Geometry check sheet. Reference: the model listing, model coordinates, mm. A direction names the side the tool comes from. Give positions to 0.01 mm unless a question says otherwise; leave off trailing zeros. Write each loop counter-clockwise with the first axis right and the second up, starting at its lowest first coordinate (ties: lowest second). Pieces come first, ordered by that corner, then holes. Notation, with made-up numbers: (11, 68) - (32, 68) arc R26 cw to (32, 91) - close; hole circle Ø3 at (11.5, -18). An arc over 180 degrees is marked (long way). Use a Markdown table: item, result.
```python
from build123d import *

# Parameters (mm, degrees)
SKETCH1_R           = 2.286
BOSS_EXTRUDE1_DEPTH = 6.35
FILLET1_R           = 3.81


with BuildPart() as part:
    # Sketch1 → Boss-Extrude1 (new body)
    with BuildSketch(Plane.XY):
        Polygon((-6.35, -6.35), (-6.35, 25.4), (6.35, 25.4), (6.35, 6.35), (31.75, 6.35), (31.75, -6.35), align=None)
        Circle(SKETCH1_R, mode=Mode.SUBTRACT)
        with Locations((12.7, 0)):
            Circle(SKETCH1_R, mode=Mode.SUBTRACT)
        with Locations((25.4, 0)):
            Circle(SKETCH1_R, mode=Mode.SUBTRACT)
        with Locations((0, 19.05)):
            Circle(SKETCH1_R, mode=Mode.SUBTRACT)
    extrude(amount=BOSS_EXTRUDE1_DEPTH)

    # Fillet1
    fillet1_edges = [part.edges().sort_by_distance(p)[0] for p in [
        (-6.35, -6.35, 3.175),
        (-6.35, 25.4, 3.175),
        (6.35, 25.4, 3.175),
        (6.35, 6.35, 3.175),
        (31.75, 6.35, 3.175),
        (31.75, -6.35, 3.175),
    ]]
    fillet(fillet1_edges, radius=FILLET1_R)


solid = part.part
```
1) Material ranges on L1, parallel to Y at x = 0, z = 3.5; L2, parallel to Y at x = 12.7, z = 5; L3, parallel to X at y = 1.5, z = 6.25, recorded low to high. Write a range as from..to.
Working result:
| item | result |
|---|---|
| L1 | y = -6.35..-2.29, 2.29..16.76, 21.34..25.4 |
| L2 | y = -6.35..-2.29, 2.29..6.35 |
| L3 | x = -6.35..-1.73, 1.73..10.97, 14.43..23.67, 27.13..31.75 |
2) Section check C-C on y = 0. Record the boundary of the cut face in (x, z).
Working result:
| item | result |
|---|---|
| outline | (-6.35, 0) - (-2.29, 0) - (-2.29, 6.35) - (-6.35, 6.35) - close; (2.29, 0) - (10.41, 0) - (10.41, 6.35) - (2.29, 6.35) - close; (14.99, 0) - (23.11, 0) - (23.11, 6.35) - (14.99, 6.35) - close; (27.69, 0) - (31.75, 0) - (31.75, 6.35) - (27.69, 6.35) - close |
3) Section check D-D on z = 3.75. Record the boundary of the cut face in (x, y), then the cut area to 3 significant figures.
Working result:
| item | result |
|---|---|
| outline | (-6.35, -2.54) arc R3.81 ccw to (-2.54, -6.35) - (27.94, -6.35) arc R3.81 ccw to (31.75, -2.54) - (31.75, 2.54) arc R3.81 ccw to (27.94, 6.35) - (10.16, 6.35) arc R3.81 cw to (6.35, 10.16) - (6.35, 21.59) arc R3.81 ccw to (2.54, 25.4) - (-2.54, 25.4) arc R3.81 ccw to (-6.35, 21.59) - close; hole circle Ø4.57 at (0, 0); hole circle Ø4.57 at (0, 19.05); hole circle Ø4.57 at (12.7, 0); hole circle Ø4.57 at (25.4, 0) |
| area | 648 mm² |
4) Mould release check, pull along X, two halves, no side actions. Record for faces 1 (the cylindrical face through (30.664, 5.204, 3.219)), 2 (the flat face through (9, 6, 6.35)), 3 (the cylindrical face through (-0.298, 21.317, 3.131)): pulls with the +X half, pulls with the -X half, needs draft (parallel to the pull), parting line crosses it, or undercut.
Working result:
| item | result |
|---|---|
| face 1 | pulls with the +X half |
| face 2 | needs draft |
| face 3 | undercut |
5) Depth check by flat-ended pin: P1, Ø1.9, axis at y = 18.5, z = 4.5, coming from the +X side; P2, Ø3, axis at x = 25.5, z = 4, coming from the +Y side. Enter the tip coordinate at first touch or a pass-through.
Working result:
| item | result |
|---|---|
| P1 | stops at x = 6.35 |
| P2 | stops at y = 6.35 |
6) Set-up check for faces 4 (the flat face through (19, 6.35, 3)), 5 (the cylindrical face through (14.8, -0.9, 3.1)): record each of +Z, -Z, +X, -X, +Y, -Y from which the full face is reachable in a straight line by a thin tool's end or side.
Working result:
| item | result |
|---|---|
| face 4 | +Z, -Z, +X, +Y |
| face 5 | +Z, -Z |
7) Section check A-A on x = 12.7. Record the boundary of the cut face in (y, z), then the cut area to 3 significant figures.
Working result:
| item | result |
|---|---|
| outline | (-6.35, 0) - (-2.29, 0) - (-2.29, 6.35) - (-6.35, 6.35) - close; (2.29, 0) - (6.35, 0) - (6.35, 6.35) - (2.29, 6.35) - close |
| area | 51.6 mm² |
